from build123d import *

# Parameters (mm, degrees)
F0_W     = 88.9
F0_H     = 28.575
F1_DEPTH = 12.7
F3_DEPTH = 6.35
F4_R     = 5.08
F6_DEPTH = 6.35
F7_R     = 3.175
F8_DEPTH = 25.4


with BuildPart() as f1:
    # F0 (on Top) → F1 (new body)
    with BuildSketch(Plane.XY):
        Rectangle(F0_W, F0_H)
    extrude(amount=F1_DEPTH)

    # F2 (on face) → F3 (cut)
    with BuildSketch(Plane.XY.offset(12.7)):
        with BuildLine():
            Line((25.4, 7.9375), (-25.4, 7.9375))
            ThreePointArc((-25.4, 7.9375), (-26.298026, 7.565526), (-26.67, 6.6675))
            Line((-26.67, 6.6675), (-26.67, 6.0325))
            ThreePointArc((-26.67, 6.0325), (-26.298026, 5.134474), (-25.4, 4.7625))
            Line((-25.4, 4.7625), (25.4, 4.7625))
            ThreePointArc((25.4, 4.7625), (26.298026, 5.134474), (26.67, 6.0325))
            Line((26.67, 6.0325), (26.67, 6.6675))
            ThreePointArc((26.67, 6.6675), (26.298026, 7.565526), (25.4, 7.9375))
        make_face()
    extrude(amount=-F3_DEPTH, mode=Mode.SUBTRACT)

    # F4
    f4_edges = [f1.edges().sort_by_distance(p)[0] for p in [
        (44.45, -14.2875, 6.35),
        (44.45, 14.2875, 6.35),
        (-44.45, -14.2875, 6.35),
        (-44.45, 14.2875, 6.35),
    ]]
    fillet(f4_edges, radius=F4_R)

    # F5 (on face) → F6 (cut)
    with BuildSketch(Plane(origin=(0, 0, 0), x_dir=(1, 0, 0), z_dir=(0, 0, -1))):
        with BuildLine():
            Line((16.002, 7.9375), (-16.002, 7.9375))
            ThreePointArc((-16.002, 7.9375), (-18.157261, 7.044761), (-19.05, 4.8895))
            Line((-19.05, 4.8895), (-19.05, 4.6355))
            ThreePointArc((-19.05, 4.6355), (-18.157261, 2.480239), (-16.002, 1.5875))
            Line((-16.002, 1.5875), (16.002, 1.5875))
            ThreePointArc((16.002, 1.5875), (18.157261, 2.480239), (19.05, 4.6355))
            Line((19.05, 4.6355), (19.05, 4.8895))
            ThreePointArc((19.05, 4.8895), (18.157261, 7.044761), (16.002, 7.9375))
        make_face()
    extrude(amount=-F6_DEPTH, mode=Mode.SUBTRACT)

    # F7 (on face) → F8 (cut)
    with BuildSketch(Plane.XY.offset(12.7)):
        with Locations((-34.925, 0)):
            Circle(F7_R)
        with Locations((34.925, 0)):
            Circle(F7_R)
    extrude(amount=-F8_DEPTH, mode=Mode.SUBTRACT)


solid = f1.part
Geometry check sheet. Reference: the model listing, model coordinates, mm. A direction names the side the tool comes from. Coordinates: 2 decimals unless noted, no trailing zeros. Order: outer loops, then holes, each group sorted by start corner. A loop starts at its lowest first (then second) coordinate and runs counter-clockwise, first axis right, second up. Notation, with made-up numbers: (54.5, -22) -> (66.5, -22) arc R26 cw to (66.5, -8) -> close; hole circle Ø3 at (33.25, 7). An arc over 180 degrees is marked (long way). Use a Markdown table: item, result. Add a question column.
1. Mould release check, pull along Y, two halves, no side actions. Record for faces 1 (the face through (0, 7.938, 10)), 2 (the face through (42.92, -12.84, 6.44)), 3 (the face through (-44.45, 0, 6)): pulls with the +Y half, pulls with the -Y half, needs draft (parallel to the pull), parting line crosses it, or undercut.
2. Set-up check for faces 4 (the face through (0, 6, 6.35)), 5 (the face through (0, -5, 6.35)), 6 (the face through (-43, -12.76, 6.44)): record each of +Z, -Z, +X, -X, +Y, -Y from which the full face is reachable in a straight line by a thin tool's end or side.
3. Go/stop test with flat-tipped pins: pin 1 Ø5 at (x, y) = (-6.5, -5) entering from -Z; pin 2 Ø2.5 at (x, y) = (-9.5, 7) entering from +Z. Record where each tip stops, or that it passes through.
4. Cross-section at C-C (x = 5). Enter the section's corners in (y, z), and give its area (3 significant figures).
5. Cross-section at A-A (z = 1.5). Give the number of separate pieces and of enclosed holes in the cut face, and give its area (3 significant figures).
6. Material ranges on L1, parallel to Y at x = -6, z = 6.25; L2, parallel to Y at x = 3, z = 7; L3, parallel to X at y = 0.5, z = 11.75, recorded low to high.
7. Cross-section at B-B (y = 0). Enter the section's corners in (x, z), and give its area (3 significant figures).
Filled sheet:
| question | item | result |
|---|---|---|
| 1 | face 1 | undercut |
| 1 | face 2 | pulls with the -Y half |
| 1 | face 3 | needs draft |
| 2 | face 4 | +Z |
| 2 | face 5 | -Z |
| 2 | face 6 | +Z, -Z, -X, -Y |
| 3 | pin 1 | z = 6.35 |
| 3 | pin 2 | z = 12.7 |
| 4 | outline | (-14.29, 0) -> (-7.94, 0) -> (-7.94, 6.35) -> (-1.59, 6.35) -> (-1.59, 0) -> (14.29, 0) -> (14.29, 12.7) -> (7.94, 12.7) -> (7.94, 6.35) -> (4.76, 6.35) -> (4.76, 12.7) -> (-14.29, 12.7) -> close |
| 4 | area | 302 mm2 |
| 5 | separate pieces | 1 |
| 5 | enclosed holes | 3 |
| 5 | area | 2,220 mm2 |
| 6 | L1 | -14.29 to -7.94, -1.59 to 14.29 |
| 6 | L2 | -14.29 to 4.76, 7.94 to 14.29 |
| 6 | L3 | -44.45 to -38.06, -31.79 to 31.79, 38.06 to 44.45 |
| 7 | outline | (-44.45, 0) -> (-38.1, 0) -> (-38.1, 12.7) -> (-44.45, 12.7) -> close; (-31.75, 0) -> (31.75, 0) -> (31.75, 12.7) -> (-31.75, 12.7) -> close; (38.1, 0) -> (44.45, 0) -> (44.45, 12.7) -> (38.1, 12.7) -> close |
| 7 | area | 968 mm2 |
